from build123d import *

# Parameters (mm, degrees)
ESBO_O1_W                = 13
ESBO_O1_H                = 14.8
ESBO_O1_W_2              = 13.26
ESBO_O1_H_2              = 2
ESBO_O1_W_3              = 2
ESBO_O1_H_3              = 6.93625866
ESBO_O1_W_4              = 12.96
RESSALTO_EXTRUS_O1_DEPTH = 2


with BuildPart() as part:
    # Esboço1 → Ressalto-extrusão1 (new body)
    with BuildSketch(Plane.XY):
        Polygon((-12.744415021, 9.596420323), (-15.664415021, 9.596420323), (-15.664415021, 7.212009238), (-15.664415021, -0.487990763), (-15.664415021, -7.424249423), (-15.664415021, -15.124249427), (-15.664415021, -18.903579677), (-12.894415021, -18.903579677), (-5.894415021, -18.903579677), (7.065584979, -18.903579677), (14.065584979, -18.903579677), (16.835584979, -18.903579677), (16.835584979, -15.124249427), (16.835584979, -7.424249423), (16.835584979, -0.487990763), (16.835584979, 7.212009238), (16.835584979, 9.596420323), (13.915584979, 9.596420323), (7.215584979, 9.596420323), (-6.044415021, 9.596420323), align=None)
        with Locations((0.585584979, -4.653579677)):
            Rectangle(ESBO_O1_W, ESBO_O1_H, mode=Mode.SUBTRACT)
        Polygon((13.915584979, 11.596420323), (13.915584979, 9.596420323), (16.835584979, 9.596420323), (16.835584979, 7.212009238), (18.835584979, 7.212009238), (18.835584979, 11.596420323), align=None)
        with Locations((0.585584979, 10.596420323)):
            Rectangle(ESBO_O1_W_2, ESBO_O1_H_2)
        Polygon((-15.664415021, 7.212009238), (-15.664415021, 9.596420323), (-12.744415021, 9.596420323), (-12.744415021, 11.596420323), (-17.664415021, 11.596420323), (-17.664415021, 7.212009238), align=None)
        with Locations((-16.664415021, -3.956120093)):
            Rectangle(ESBO_O1_W_3, ESBO_O1_H_3)
        Polygon((-15.664415021, -18.903579677), (-15.664415021, -15.124249427), (-17.664415021, -15.124249427), (-17.664415021, -20.903579677), (-12.894415021, -20.903579677), (-12.894415021, -18.903579677), align=None)
        with Locations((0.585584979, -19.903579677)):
            Rectangle(ESBO_O1_W_4, ESBO_O1_H_2)
        Polygon((18.835584979, -15.124249427), (16.835584979, -15.124249427), (16.835584979, -18.903579677), (14.065584979, -18.903579677), (14.065584979, -20.903579677), (18.835584979, -20.903579677), align=None)
        with Locations((17.835584979, -3.956120093)):
            Rectangle(ESBO_O1_W_3, ESBO_O1_H_3)
    extrude(amount=RESSALTO_EXTRUS_O1_DEPTH)


solid = part.part
Verification items for the finished model (mm, model axes). A direction names the side the tool comes from. Give positions to 0.01 mm unless a question says otherwise; leave off trailing zeros. Write each loop counter-clockwise with the first axis right and the second up, starting at its lowest first coordinate (ties: lowest second). Pieces come first, ordered by that corner, then holes. Notation, with made-up numbers: M 65.25,38 L 85.25,38 A23 cw 85.25,63 Z; hole C -32,-15.75 d9. An arc over 180 degrees is marked long. Use CSV: the item, a comma, the result in double quotes.
1) Cross-section at A-A (y = 1). Enter the section's corners in (x, z).
Final values:
outline,"M -15.66,0 L -5.91,0 L -5.91,2 L -15.66,2 Z; M 7.09,0 L 16.84,0 L 16.84,2 L 7.09,2 Z"
2) Cross-section at B-B (x = 4). Enter the section's corners in (y, z).
Final values:
outline,"M -20.9,0 L -12.05,0 L -12.05,2 L -20.9,2 Z; M 2.75,0 L 11.6,0 L 11.6,2 L 2.75,2 Z"
3) Material ranges on line 1 along Y through (x, z) = (17, 0.1); line 2 along X through (y, z) = (-1, 1); line 3 along Y through (x, z) = (2.5, 0.65), recorded low to high.
Final values:
line 1,"-20.9 to -15.12, -7.42 to -0.49, 7.21 to 11.6"
line 2,"-17.66 to -5.91, 7.09 to 18.84"
line 3,"-20.9 to -12.05, 2.75 to 11.6"
4) Release check for a two-part mould opening along Y. For faces 1 (the face through (11, 9.596, 1)), 2 (the face through (7.086, -5, 1)), 3 (the face through (-5.894, -20, 1)) record: released by +Y, released by -Y, zero draft, split by the parting line, or undercut.
Final values:
face 1,"released by +Y"
face 2,"undercut"
face 3,"zero draft"
5) Go/stop test with flat-tipped pins: pin 1 Ø0.6 at (y, z) = (-10, 1) entering from +X; pin 2 Ø1 at (y, z) = (4, 1) entering from -X. Record where each tip stops, or that it passes through.
Final values:
pin 1,"x = 16.84"
pin 2,"x = -15.66"
6) Access from +Z, -Z, +X, -X, +Y, -Y to the whole of each face (thin tool, end or side, straight path). Record for faces 4 (the face through (16.836, -11, 1)), 5 (the face through (-9, 9.596, 1)), 6 (the face through (-5.914, -5, 1)), 7 (the face through (-15.664, 3, 1)), 8 (the face through (7.066, -20, 1)).
Final values:
face 4,"+Z, -Z, +X"
face 5,"+Z, -Z, +Y"
face 6,"+Z, -Z"
face 7,"+Z, -Z, -X"
face 8,"+Z, -Z, -Y"
